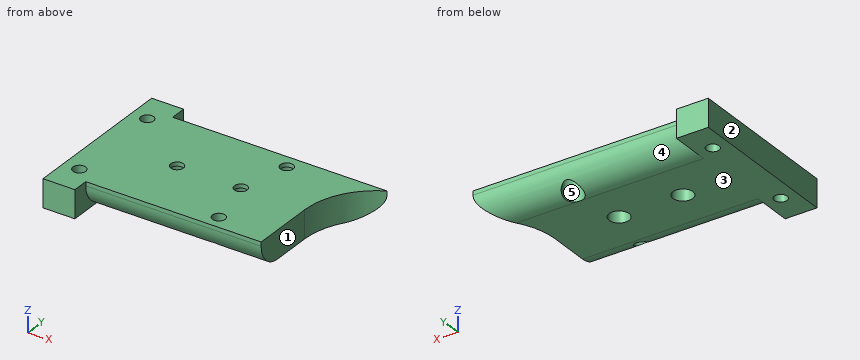
```python
from build123d import *

# Parameters (mm, degrees)
SKETCH1_W           = 4
SKETCH1_H           = 2
BOSS_EXTRUDE1_DEPTH = 3.5
SKETCH2_R           = 0.8
SCREW_HOLES_DEPTH   = 43.383720665
SKETCH3_R           = 1.25
SCREW_HEADS_DEPTH   = 3
FILLET1_R           = 3


with BuildPart() as part:
    # Sketch1 → Boss-Extrude1 (new body)
    with BuildSketch(Plane.XY):
        with BuildLine():
            Line((10.161255894, 0), (36.161255894, 0))
            ThreePointArc((36.161255894, 0), (37.476597455, 4.684658438), (41.038150268, 8))
            Line((41.038150268, 8), (14.161255894, 8))
            Line((14.161255894, 8), (10.161255894, 8))
            Line((10.161255894, 8), (10.161255894, 0))
        make_face()
        Polygon((36.161255894, -8), (36.161255894, 0), (10.161255894, 0), (10.161255894, -8), (14.161255894, -8), align=None)
        with Locations((12.161255894, 9)):
            Rectangle(SKETCH1_W, SKETCH1_H)
        with Locations((12.161255894, -9)):
            Rectangle(SKETCH1_W, SKETCH1_H)
    extrude(amount=BOSS_EXTRUDE1_DEPTH)

    # Sketch2 → Screw Holes (cut, through all)
    with BuildSketch(Plane.XY):
        with Locations((20.161255894, 0)):
            Circle(SKETCH2_R)
        with Locations((12.161255894, -6.25)):
            Circle(SKETCH2_R)
        with Locations((29.661255894, 6.25)):
            Circle(SKETCH2_R)
        with Locations((29.661255894, -6.25)):
            Circle(SKETCH2_R)
        with Locations((12.161255894, 6.25)):
            Circle(SKETCH2_R)
        with Locations((28.161255894, 0)):
            Circle(SKETCH2_R)
    extrude(amount=SCREW_HOLES_DEPTH, mode=Mode.SUBTRACT)

    # Sketch3 → Screw Heads (cut)
    with BuildSketch(Plane.XY):
        with Locations((20.161255894, 0)):
            Circle(SKETCH3_R)
        with Locations((29.661255894, 6.25)):
            Circle(SKETCH3_R)
        with Locations((28.161255894, 0)):
            Circle(SKETCH3_R)
    extrude(amount=SCREW_HEADS_DEPTH, mode=Mode.SUBTRACT)

    # Fillet1
    # the kernel refuses this fillet: 3 mm, written as the material it takes off along each edge
    with BuildSketch(Plane(origin=(48.538150268, 8, 0), x_dir=(0, 0, 1), z_dir=(-1, 0, 0))) as fillet1_piece_1:
        with BuildLine():
            CenterArc((FILLET1_R, -FILLET1_R), FILLET1_R, 90, 90)
            Line((0, -FILLET1_R), (0, 0))
            Line((0, 0), (FILLET1_R, 0))
        make_face()
    extrude(amount=34.376894374, mode=Mode.SUBTRACT)
    with BuildSketch(Plane(origin=(14.161255894, -8, 0), x_dir=(0, 0, 1), z_dir=(1, 0, 0))) as fillet1_piece_2:
        with BuildLine():
            CenterArc((FILLET1_R, -FILLET1_R), FILLET1_R, 90, 90)
            Line((0, -FILLET1_R), (0, 0))
            Line((0, 0), (FILLET1_R, 0))
        make_face()
    extrude(amount=29.5, mode=Mode.SUBTRACT)


solid = part.part
```
CAD build for the part. Positions are in the model's coordinates, mm. Face numbers are marked on the shaded views. A direction names the side the tool comes from. Round coordinates to 2 decimals unless told otherwise and drop trailing zeros. Order: outer loops, then holes, each group sorted by start corner. A loop starts at its lowest first (then second) coordinate and runs counter-clockwise, first axis right, second up. Notation, with made-up numbers: (-32, -19) - (9, -19) arc R29 ccw to (9, 15) - close; hole circle Ø7 at (53, 83). An arc over 180 degrees is marked (long way). Answer in a Markdown table with one row per item. Add a question column.
(1) 3-axis set-ups, long thin cutter, end or side, ignore diameter. For the marked faces 1 and 2: which of +Z, -Z, +X, -X, +Y, -Y reach the whole face in a straight line?
(2) Band-saw the part on A-A on y = -6.25. List the corners of the cut face in (x, z).
(3) Mould opens along Y. For the marked faces 3, 4 and 5 say: +Y half, -Y half, draft (parallel to the pull), parting line (faces both ways), or undercut.
(4) Band-saw the part on C-C on z = 1.65. List the corners of the cut face in (x, y), and give its area (3 significant figures).
(5) Band-saw the part on B-B on x = 12. List the corners of the cut face in (y, z), and give its area (3 significant figures).
(6) Band-saw the part on D-D on x = 32. List the corners of the cut face in (y, z).
(7) Drop flat-ended pins along their axis: pin 1 Ø0.6 at (x, z) = (29, 3.5) entering from +Y; pin 2 Ø2 at (x, y) = (30, 7) entering from -Z; pin 3 Ø1 at (y, z) = (-7, 1) entering from +X. Give the stop position or say it passes through.
(8) Probe L1, parallel to X at y = -1, z = 2.75; L2, parallel to X at y = 6.25, z = 3.4; L3, parallel to Y at x = 18, z = 3.2. List the from-to ranges inside material, lowest first. Write a range as [from, to].
Data:
| question | item | result |
|---|---|---|
| 1 | face 1 | +Z, -Z, +X, -Y |
| 1 | face 2 | +Z, -Z, -X, +Y, -Y |
| 2 | outline | (10.16, 0) - (11.36, 0) - (11.36, 3.5) - (10.16, 3.5) - close; (12.96, 0) - (14.16, 0) - (14.16, 0.27) - (28.86, 0.27) - (28.86, 3.5) - (12.96, 3.5) - close; (30.46, 0.27) - (36.16, 0.27) - (36.16, 3.5) - (30.46, 3.5) - close |
| 3 | face 3 | draft |
| 3 | face 4 | +Y half |
| 3 | face 5 | undercut |
| 4 | outline | (10.16, -10) - (14.16, -10) - (14.16, -7.68) - (36.16, -7.68) - (36.16, 0) arc R9 cw to (40.47, 7.68) - (14.16, 7.68) - (14.16, 10) - (10.16, 10) - close; hole circle Ø1.6 at (12.16, -6.25); hole circle Ø1.6 at (12.16, 6.25); hole circle Ø2.5 at (20.16, 0); hole circle Ø2.5 at (28.16, 0); hole circle Ø2.5 at (29.66, 6.25); hole circle Ø1.6 at (29.66, -6.25) |
| 4 | area | 407 mm^2 |
| 5 | outline | (-10, 0) - (-7.03, 0) - (-7.03, 3.5) - (-10, 3.5) - close; (-5.47, 0) - (5.47, 0) - (5.47, 3.5) - (-5.47, 3.5) - close; (7.03, 0) - (10, 0) - (10, 3.5) - (7.03, 3.5) - close |
| 5 | area | 59.0 mm^2 |
| 6 | outline | (-8, 3) arc R3 ccw to (-5, 0) - (5, 0) arc R3 ccw to (8, 3) - (8, 3.5) - (-8, 3.5) - close |
| 7 | pin 1 | stops at y = 8 |
| 7 | pin 2 | stops at z = 0.42 |
| 7 | pin 3 | stops at x = 36.16 |
| 8 | L1 | x = [10.16, 19.41], [20.91, 27.41], [28.91, 36.16] |
| 8 | L2 | x = [10.16, 11.36], [12.96, 28.86], [30.46, 38.69] |
| 8 | L3 | y = [-8, 8] |
